For this review, take the finished solid that the model builds, in its own axes (mm). Give positions to 0.01 mm unless a question says otherwise; leave off trailing zeros. Order: outer loops, then holes, each group sorted by start corner. A loop starts at its lowest first (then second) coordinate and runs counter-clockwise, first axis right, second up.
from build123d import *

# Parameters (mm, degrees)
SKETCH_1_W      = 94
SKETCH_1_H      = 64
SKETCH_1_R      = 10
SKETCH_1_R_2    = 1.7
SKETCH_1_R_3    = 1.6
EXTRUDE_1_DEPTH = 2


with BuildPart() as part:
    # 草图1 → 凸台-拉伸1 (new, symmetric)
    with BuildSketch(Plane.XY):
        with Locations((-45, 102)):
            Rectangle(SKETCH_1_W, SKETCH_1_H)
        with Locations((-70, 92)):
            Circle(SKETCH_1_R, mode=Mode.SUBTRACT)
        with Locations((-35, 118)):
            Circle(SKETCH_1_R_2, mode=Mode.SUBTRACT)
        with Locations((-9, 104.5)):
            Circle(SKETCH_1_R_2, mode=Mode.SUBTRACT)
        with Locations((-37, 104.5)):
            Circle(SKETCH_1_R_2, mode=Mode.SUBTRACT)
        with Locations((-88, 74)):
            Circle(SKETCH_1_R_3, mode=Mode.SUBTRACT)
        with Locations((-2, 74)):
            Circle(SKETCH_1_R_3, mode=Mode.SUBTRACT)
        with Locations((-45, 108)):
            Circle(SKETCH_1_R_3, mode=Mode.SUBTRACT)
    extrude(amount=EXTRUDE_1_DEPTH, both=True)


solid = part.part
1) We need section A-A on y = 92. Give the boundary of the cut face in (x, z), then the cut area to 3 significant figures.
Answer sheet:
outline: (-92, -2) - (-80, -2) - (-80, 2) - (-92, 2) - close; (-60, -2) - (2, -2) - (2, 2) - (-60, 2) - close
area: 296 mm2
2) We need section C-C on z = 0.5. Give the boundary of the cut face in (x, y), then the cut area to 3 significant figures.
Answer sheet:
outline: (-92, 70) - (2, 70) - (2, 134) - (-92, 134) - close; hole circle Ø3.2 at (-88, 74); hole circle Ø20 at (-70, 92); hole circle Ø3.2 at (-45, 108); hole circle Ø3.4 at (-37, 104.5); hole circle Ø3.4 at (-35, 118); hole circle Ø3.4 at (-9, 104.5); hole circle Ø3.2 at (-2, 74)
area: 5,650 mm2
3) Draft analysis for pull direction X (two halves, no side actions). For faces 1 (the face through (-46, 134, 0)), 2 (the face through (2, 102, 0)), 3 (the face through (-77.37, 98.76, -0.03)), 4 (the face through (-92, 102, 0)), state which applies: +X half, -X half, draft (parallel to the pull), parting line (faces both ways), or undercut.
Answer sheet:
face 1: draft
face 2: +X half
face 3: undercut
face 4: -X half
4) We need section B-B on x = -2. Give the boundary of the cut face in (y, z), then the cut area to 3 significant figures.
Answer sheet:
outline: (70, -2) - (72.4, -2) - (72.4, 2) - (70, 2) - close; (75.6, -2) - (134, -2) - (134, 2) - (75.6, 2) - close
area: 243 mm2
5) We need section D-D on y = 104.5. Give the boundary of the cut face in (x, z).
Answer sheet:
outline: (-92, -2) - (-38.7, -2) - (-38.7, 2) - (-92, 2) - close; (-35.3, -2) - (-10.7, -2) - (-10.7, 2) - (-35.3, 2) - close; (-7.3, -2) - (2, -2) - (2, 2) - (-7.3, 2) - close
6) Clearance check with a flat-ended pin moving along its axis: pin 1 (3 mm diameter, centred on x = -45, y = 108, fed in from -Z). State where the tip first meets the part, or that it passes through.
Answer sheet:
pin 1: passes through
7) To check wall thickness, follow line 1 (X direction, y = 104.5, z = -0.1); line 2 (X direction, y = 74, z = -0.05); line 3 (Y direction, x = -35, z = -1.8). State the ranges of each line that lie inside material, in increasing order.
Answer sheet:
line 1: x = -92 to -38.7, -35.3 to -10.7, -7.3 to 2
line 2: x = -92 to -89.6, -86.4 to -3.6, -0.4 to 2
line 3: y = 70 to 116.3, 119.7 to 134
